The listing builds one solid part. Answer for the finished solid, in the listing's coordinates (mm). A direction names the side the tool comes from. Give positions to 0.01 mm unless a question says otherwise; leave off trailing zeros. Loops run counter-clockwise (first coordinate to the right, second up) from the corner with the lowest first, then second, coordinate; pieces in that order, holes last. Notation, with made-up numbers: M -19,-24 L 34,-24 A8 ccw 34,-15 Z; hole C 39.5,-40 d4. An arc over 180 degrees is marked long. One line per item, written item: value. Start each with the question number.
Q1. A cutting plane is placed at D-D, the plane x = -15.5. Determine the outline of the cut face in (y, z), and give its area (4 significant figures).
Q2. A cutting plane is placed at B-B, the plane z = 0. Determine the outline of the cut face in (x, y).
Q3. Consider L1, parallel to Y at x = 16.5, z = 23.5; L2, parallel to X at y = 15, z = 21.5; L3, parallel to X at y = 35.5, z = 5.5. Determine where each line is inside the solid, lowest interval first.
Q4. A cutting plane is placed at A-A, the plane x = 0. Determine the outline of the cut face in (y, z), and give its area (3 significant figures).
Q5. A cutting plane is placed at C-C, the plane y = 5.5. State how many separate pieces and enclosed holes the cut face has, and give its area (3 significant figures).
Q6. For faces 1 (the flat face through (22, 7.5, -22)), 2 (the cylindrical face through (6.2, 35.03, -9.72)), 3 (the flat face through (25, 13, 0)), determine the directions among +Z, -Z, +X, -X, +Y, -Y from which every point of the face is accessible in a straight line to the end or side of a thin tool.
Q7. Flat-ended cylindrical pins translate along their axes: pin 1 (1 mm diameter, centred on x = -6.5, z = -0.5, fed in from +Y); pin 2 (0.9 mm diameter, centred on x = -21.5, z = -22, fed in from -Y); pin 3 (10 mm diameter, centred on x = -15.5, z = 16.5, fed in from +Y). Find the tip coordinate at first contact, or state that the pin passes through.
Q8. The mould has two halves that part along Z. Classify faces 4 (the flat face through (-22, 7.5, -22)), 5 (the cylindrical face through (23.01, 3.7, 20.89)), 6 (the flat face through (0, 42.32, 0)), 7 (the flat face through (0, 13, 25)): +Z half, -Z half, draft (parallel to the pull), parting line (faces both ways), or undercut.
from build123d import *

# Parameters (mm, degrees)
SKETCH3_W           = 50
SKETCH3_H           = 50
BOSS_EXTRUDE1_DEPTH = 26.5
SKETCH4_R           = 1.5
CUT_EXTRUDE1_DEPTH  = 7.5
VARFILLET1_START    = -1
VARFILLET1_DEPTH    = 28


with BuildPart() as part:
    # Sketch3 → Boss-Extrude1 (new body)
    with BuildSketch(Plane(origin=(0, 0, 0), x_dir=(1, 0, 0), z_dir=(0, 1, 0))):
        Rectangle(SKETCH3_W, SKETCH3_H)
    extrude(amount=BOSS_EXTRUDE1_DEPTH)

    # Sketch4 → Cut-Extrude1 (cut)
    with BuildSketch(Plane(origin=(0, 0, 0), x_dir=(1, 0, 0), z_dir=(0, 1, 0))):
        with Locations(Location((22.000213283, 22.000213283, 0), (0, 0, 270))):
            Circle(SKETCH4_R)
        with Locations(Location((22.000213283, -22.000213283, 0), (0, 0, 270))):
            Circle(SKETCH4_R)
        with Locations(Location((-22.000213283, -22.000213283, 0), (0, 0, 270))):
            Circle(SKETCH4_R)
        with Locations(Location((-22.000213283, 22.000213283, 0), (0, 0, 270))):
            Circle(SKETCH4_R)
    extrude(amount=CUT_EXTRUDE1_DEPTH, mode=Mode.SUBTRACT)

    # Sketch6 → Revolve1 (revolve)
    with BuildSketch(Plane.XY):
        with BuildLine():
            Line((0, 42.32), (0, 26.5))
            Line((0, 26.5), (12, 26.5))
            Line((12, 26.5), (12, 31.5))
            Line((12, 31.5), (11.530705563, 32.5))
            Line((11.530705563, 32.5), (11.530705563, 37.5))
            ThreePointArc((11.530705563, 37.5), (6.71772817, 40.886032515), (1.010390364, 42.32))
            Line((1.010390364, 42.32), (0, 42.32))
        make_face()
    revolve(axis=Axis((0, 26.5, 0), (0, 1, 0)))

    # VarFillet1: read off the stored shape, not the designer's step
    # VarFillet1 outline → VarFillet1 (cut)
    with BuildSketch(Plane(origin=(0, 0, 0), x_dir=(1, 0, 0), z_dir=(0, 1, 0)).offset(VARFILLET1_START)):
        with BuildLine():
            Line((-25, -25), (-20, -25))
            add(Edge.make_bspline(
                [(-20, -25), (-25, -25), (-25, -20)],
                knots=[0, 0, 0, 1, 1, 1], degree=2, weights=[1, 0.707106781, 1]))
            Line((-25, -20), (-25, -25))
        make_face()
        with BuildLine():
            add(Edge.make_bspline(
                [(25, -20), (25, -25), (20, -25)],
                knots=[0, 0, 0, 1, 1, 1], degree=2, weights=[1, 0.707106781, 1]))
            Line((20, -25), (25, -25))
            Line((25, -25), (25, -20))
        make_face()
        with BuildLine():
            Line((-25, 25), (-25, 20))
            add(Edge.make_bspline(
                [(-25, 20), (-25, 25), (-20, 25)],
                knots=[0, 0, 0, 1, 1, 1], degree=2, weights=[1, 0.707106781, 1]))
            Line((-20, 25), (-25, 25))
        make_face()
        with BuildLine():
            add(Edge.make_bspline(
                [(20, 25), (25, 25), (25, 20)],
                knots=[0, 0, 0, 1, 1, 1], degree=2, weights=[1, 0.707106781, 1]))
            Line((25, 20), (25, 25))
            Line((25, 25), (20, 25))
        make_face()
    extrude(amount=VARFILLET1_DEPTH, mode=Mode.SUBTRACT)


solid = part.part
Answer block:
1. outline: M 0,-25 L 26.5,-25 L 26.5,25 L 0,25 Z
1. area: 1,325 mm^2
2. outline: M -25,0 L 25,0 L 25,26.5 L 12,26.5 L 12,31.5 L 11.53,32.5 L 11.53,37.5 A16.13 ccw 1.01,42.32 L -1.01,42.32 A16.13 ccw -11.53,37.5 L -11.53,32.5 L -12,31.5 L -12,26.5 L -25,26.5 Z
3. L1: 0 to 26.5
3. L2: -24.77 to 24.77
3. L3: -10.13 to 10.13
4. outline: M 0,-25 L 26.5,-25 L 26.5,-12 L 31.5,-12 L 32.5,-11.53 L 37.5,-11.53 A16.13 ccw 42.32,-1.01 L 42.32,1.01 A16.13 ccw 37.5,11.53 L 32.5,11.53 L 31.5,12 L 26.5,12 L 26.5,25 L 0,25 Z
4. area: 1,660 mm^2
5. separate pieces: 1
5. enclosed holes: 4
5. area: 2,450 mm^2
6. face 1: -Y
6. face 2: +Y
6. face 3: +Z, -Z, +X, +Y, -Y
7. pin 1: y = 41.19
7. pin 2: y = 7.5
7. pin 3: y = 26.5
8. face 4: undercut
8. face 5: undercut
8. face 6: draft
8. face 7: +Z half
